from build123d import *

# Parameters (mm, degrees)
F2_R     = 7.9375
F3_DEPTH = 14.352


with BuildPart() as f1:
    # F0 (on Front) → F1 (revolve)
    with BuildSketch(Plane.XZ):
        Polygon((3.2512, 15.0876), (0, 15.0876), (0, 11.176), (15.875, 11.176), (15.875, 17.4625), (14.351, 17.4625), (14.351, 50.8), (3.2512, 50.8), align=None)
    revolve(axis=Axis((-0.422707, 0, 0), (1, 0, 0)))

    # F2 (on face) → F3 (cut, through all)
    with BuildSketch(Plane.YZ.offset(14.351)):
        with Locations((0, 30.988)):
            Circle(F2_R)
        with Locations((-30.988, 0)):
            Circle(F2_R)
        with Locations((0, -30.988)):
            Circle(F2_R)
        with Locations((30.988, 0)):
            Circle(F2_R)
    extrude(amount=-F3_DEPTH, mode=Mode.SUBTRACT)


solid = f1.part
Build history of the part. All positions in model axes, mm. A direction names the side the tool comes from. Round coordinates to 2 decimals unless told otherwise and drop trailing zeros. Order: outer loops, then holes, each group sorted by start corner. A loop starts at its lowest first (then second) coordinate and runs counter-clockwise, first axis right, second up. Notation, with made-up numbers: M 86,26 L 110,26 A23 ccw 110,50 Z; hole C -20.75,56.5 d9. An arc over 180 degrees is marked long. Use CSV: the item, a comma, the result in double quotes. Start each with the question number.
(1) Cut at A-A on z = 0. List the corners of the cut face in (x, y) (1 decimal).
(2) Flat gauge pins, fed straight in: P1, Ø5, axis at x = 14, z = -9, coming from the -Y side; P2, Ø20.5, axis at y = 0, z = 30.988, coming from the +X side; P3, Ø1, axis at x = 11, z = 37, coming from the +Y side. Where does each tip first touch, or does it go through?
(3) Mould opens along Y. For faces 1 (the face through (0, 6, -10)), 2 (the face through (1.603, 9.181, -11.973)), 3 (the face through (8.88, -1.72, 23.24)) say: +Y half, -Y half, draft (parallel to the pull), parting line (faces both ways), or undercut.
(4) Cut at D-D on x = 1.5. List the corners of the cut face in (y, z).
(5) Tool access for faces 4 (the face through (14.351, 22, 1)), 5 (the face through (3.251, -12, 11)), 6 (the face through (8.879, 4.267, -24.295)): list every direction of +Z, -Z, +X, -X, +Y, -Y with a clear straight run to the whole face (end or side of a thin tool).
(6) Cut at C-C on y = 26. List the corners of the cut face in (x, z), then the cut area to 3 significant figures.
(7) Drill centre lines: probe 1 along Y at (x, z) = (8.75, 0.5); probe 2 along Z at (x, y) = (11, 0); probe 3 along Z at (x, y) = (14.25, 6.5). Where is each one in solid material? Low to high.
Findings:
1,outline,"M 0,-15.1 L 3.3,-15.1 L 3.3,-23.1 L 14.4,-23.1 L 14.4,-17.5 L 15.9,-17.5 L 15.9,-11.2 L 0,-11.2 Z; M 0,11.2 L 15.9,11.2 L 15.9,17.5 L 14.4,17.5 L 14.4,23.1 L 3.3,23.1 L 3.3,15.1 L 0,15.1 Z; M 3.3,-50.8 L 14.4,-50.8 L 14.4,-38.9 L 3.3,-38.9 Z; M 3.3,38.9 L 14.4,38.9 L 14.4,50.8 L 3.3,50.8 Z"
2,P1,"stops at y = -50.38"
2,P2,"stops at x = 14.35"
2,P3,"stops at y = 35.33"
3,face 1,"draft"
3,face 2,"parting line"
3,face 3,"undercut"
4,outline,"C 0,0 d30.18; hole C 0,0 d22.35"
5,face 4,"+X"
5,face 5,"-X"
5,face 6,"+X, -X"
6,outline,"M 3.25,-43.64 L 14.35,-43.64 L 14.35,-6.17 L 3.25,-6.17 Z; M 3.25,6.17 L 14.35,6.17 L 14.35,43.64 L 3.25,43.64 Z"
6,area,"832 mm^2"
7,probe 1,"y = -50.8 to -38.91, -23.07 to -11.16, 11.16 to 23.07, 38.91 to 50.8"
7,probe 2,"z = -50.8 to -38.93, -23.05 to -11.18, 11.18 to 23.05, 38.93 to 50.8"
7,probe 3,"z = -50.38 to -35.54, -26.43 to -9.09, 9.09 to 26.43, 35.54 to 50.38"
